Read the model definition and answer for the solid it produces. Units are mm, in the model's axes. Face numbers are marked on the shaded views. Coordinates: 2 decimals unless noted, no trailing zeros. Write each loop counter-clockwise with the first axis right and the second up, starting at its lowest first coordinate (ties: lowest second). Pieces come first, ordered by that corner, then holes.
Item 1: Determine the mould class of the marked faces 1, 2 and 3 for opening direction Z: released by +Z, released by -Z, zero draft, split by the parting line, or undercut.
Item 2: Section A-A (y = 0) is taken. Give the vertices of the cut face in (x, z), then the cut area to 3 significant figures.
Item 3: Section B-B (x = 3) is taken. Give the vertices of the cut face in (y, z).
Item 4: Section C-C (x = 33) is taken. Give the vertices of the cut face in (y, z).
Item 5: Straight lines are drawn through the part: probe 1 along Z at (x, y) = (28, -0.5); probe 2 along X at (y, z) = (-1.5, -1.25); probe 3 along Y at (x, z) = (34.05, 0). For each, find the intervals that lie inside material, in ascending order.
Item 6: Each of these flat-tipped pins is pushed along its axis until it touches: P1, Ø2, axis at x = 10.5, y = -3, coming from the +Z side; P2, Ø1.6, axis at x = 8.5, y = 1, coming from the -Z side; P3, Ø1.2, axis at x = 3, y = 0, coming from the +Z side; P4, Ø1, axis at x = 22, y = -0.5, coming from the +Z side. Where does it stop, or does it pass through?
Item 7: Section D-D (x = 16) is taken. Give the vertices of the cut face in (y, z), then the cut area to 3 significant figures.
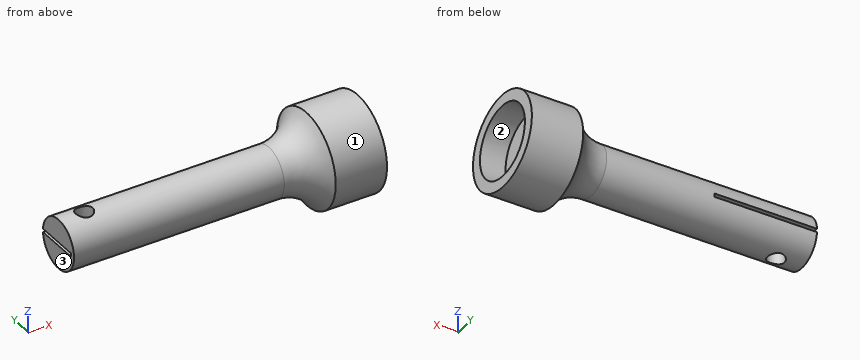
from build123d import *

# Parameters (mm, degrees)
SKETCH_1_R               = 2.9
EXTRUDE_1_DEPTH          = 35
SKETCH_2_W               = 0.4
SKETCH_2_H               = 5.450532248
CUT_EXTRUDE_1_DEPTH      = 12
CUT_EXTRUDE_2_DEPTH      = 10
CUT_EXTRUDE_2_DEPTH_BACK = 10
SKETCH_3_R               = 1
SKETCH_4_R               = 5.5
EXTRUDE_2_DEPTH          = 6
SKETCH_5_R               = 4.2
CUT_EXTRUDE_3_DEPTH      = 3
FILLET_1_R               = 5


with BuildPart() as part:
    # 草图1 → 凸台-拉伸1 (new body)
    with BuildSketch(Plane(origin=(0, 0, 0), x_dir=(0, 0, -1), z_dir=(1, 0, 0))):
        Circle(SKETCH_1_R)
    extrude(amount=EXTRUDE_1_DEPTH)

    # 草图2 → 切除-拉伸1 (cut)
    with BuildSketch(Plane.ZY):
        with Locations((0, 0.396255312)):
            Rectangle(SKETCH_2_W, SKETCH_2_H)
    extrude(amount=-CUT_EXTRUDE_1_DEPTH, mode=Mode.SUBTRACT)

    # 草图3 → 切除-拉伸2 (cut, two sides: drawn at the far end of the back side and taken through both)
    with BuildSketch(Plane(origin=(0, 0, 0.2), x_dir=(-1, 0, 0), z_dir=(0, 0, -1)).offset(-CUT_EXTRUDE_2_DEPTH_BACK)):
        with Locations(Location((-3, -0.003452386, 0), (0, 0, 270))):
            Circle(SKETCH_3_R)
    extrude(amount=CUT_EXTRUDE_2_DEPTH + CUT_EXTRUDE_2_DEPTH_BACK, mode=Mode.SUBTRACT)

    # 草图4 → 凸台-拉伸2 (add)
    with BuildSketch(Plane(origin=(35, 0, 0), x_dir=(0, 0, -1), z_dir=(1, 0, 0))):
        Circle(SKETCH_4_R)
    extrude(amount=-EXTRUDE_2_DEPTH)

    # 草图5 → 切除-拉伸3 (cut)
    with BuildSketch(Plane(origin=(35, 0, 0), x_dir=(0, 0, -1), z_dir=(1, 0, 0))):
        Circle(SKETCH_5_R)
    extrude(amount=-CUT_EXTRUDE_3_DEPTH, mode=Mode.SUBTRACT)

    # 圆角1
    # the kernel refuses this fillet: 5 mm, written as the material it adds along each edge
    with BuildSketch(Plane(origin=(29, 0, 0), x_dir=(0, 0, -1), z_dir=(0, 1, 0))) as fillet_1_piece_1:
        with BuildLine():
            CenterArc((7.9, 4.38634244), FILLET_1_R, 180, 61.314597986)
            Line((5.5, 0), (5.452, -0.087726849))
            ThreePointArc((5.452, -0.087726849), (4.2, -0.1), (2.9, -0.1))
            Line((2.9, -0.1), (2.8, 0))
            Line((2.8, 0), (2.8, 4.38634244))
            Line((2.8, 4.38634244), (2.9, 4.38634244))
        make_face()
    revolve(axis=Axis((29, 0, 0), (-1, 0, 0)))


solid = part.part
Established:
1. face 1: split by the parting line
1. face 2: undercut
1. face 3: zero draft
2. outline: (0, -2.9) - (2, -2.9) - (2, -0.2) - (0, -0.2) - close; (0, 0.2) - (2, 0.2) - (2, 2.9) - (0, 2.9) - close; (4, -2.9) - (24.61, -2.9) arc R5 cw to (29, -5.5) - (35, -5.5) - (35, -4.2) - (32, -4.2) - (32, 4.2) - (35, 4.2) - (35, 5.5) - (29, 5.5) arc R5 cw to (24.61, 2.9) - (4, 2.9) - (4, 0.2) - (12, 0.2) - (12, -0.2) - (4, -0.2) - close
2. area: 200 mm2
3. outline: (-2.33, -0.2) - (-2.33, 0.2) - (-1, 0.2) - (-1, 2.72) arc R2.9 ccw to (-1, -2.72) - (-1, -0.2) - close; (1, -2.72) arc R2.9 ccw to (2.89, -0.2) - (1, -0.2) - close; (1, 0.2) - (2.89, 0.2) arc R2.9 ccw to (1, 2.72) - close
4. outline: circle Ø11 at (0, 0); hole circle Ø8.4 at (0, 0)
5. probe 1: z = -4.19 to 4.19
5. probe 2: x = 0 to 32
5. probe 3: y = -5.5 to -4.2, 4.2 to 5.5
6. P1: stops at z = 2.1
6. P2: stops at z = -2.89
6. P3: passes through
6. P4: stops at z = 2.9
7. outline: circle Ø5.8 at (0, 0)
7. area: 26.4 mm2
